Geometry: final body of the model. Coordinates: model frame, mm. Face numbers are marked on the shaded views. A direction names the side the tool comes from. Give positions to 0.01 mm unless a question says otherwise; leave off trailing zeros. Write each loop counter-clockwise with the first axis right and the second up, starting at its lowest first coordinate (ties: lowest second). Pieces come first, ordered by that corner, then holes. Notation, with made-up numbers: (-10, 83) - (4, 83) arc R14 cw to (4, 103) - close; hole circle Ø5 at (-10.5, 24). An arc over 180 degrees is marked (long way). Use CSV: the item, a comma, the result in double quotes. Start each with the question number.
(1) Section D-D on y = 220. Output: boundary loops of the cut face in (x, z), and give its area (3 significant figures).
(2) Section B-B on z = 62. Output: boundary loops of the cut face in (x, y).
(3) Line query: probe 1 along Z at (x, y) = (0, 14.75); probe 2 along Y at (x, z) = (0, -1); probe 3 along Y at (x, z) = (0, 2.75). Output: solid intervals per line, ascending. Write a range as [from, to].
(4) Section C-C on y = 15.5. Output: boundary loops of the cut face in (x, z).
(5) Reachability of the marked faces 1 and 2 from +Z, -Z, +X, -X, +Y, -Y: full face, straight path, thin tool, end or side. Return the list, or none.
(6) First-contact query: pin 1 Ø4 at (x, z) = (2.5, 38) entering from -Y; pin 2 Ø12 at (x, y) = (0, 182) entering from +Z; pin 3 Ø4 at (x, z) = (-4.5, 33) entering from -Y; pin 4 Ø10 at (y, z) = (121.5, -1) entering from -X. Flat tips, straight axial feed; report the tip coordinate or a pass-through.
(7) Section A-A on y = 100. Output: boundary loops of the cut face in (x, z).
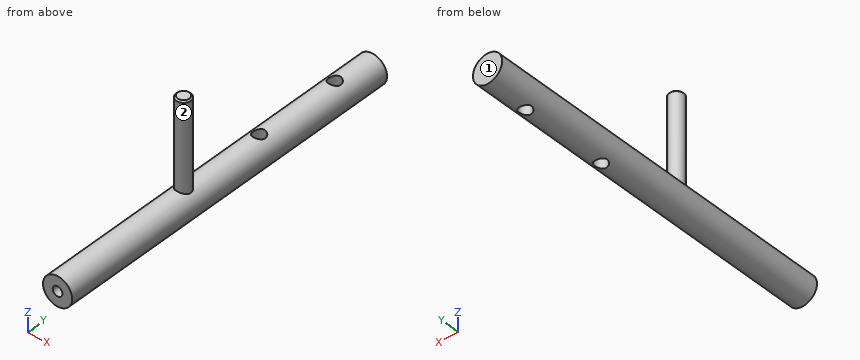
Autodesk Inventor part; units mm, degrees
ref_plane "Arbeitsebene1" through (0, 0, 3.5) normal (0, 0, 1) x (1, 0, 0)
ref_plane "YZ Plane" through (0, 0, 0) normal (1, 0, 0) x (0, 1, 0)
ref_plane "XZ Plane" through (0, 0, 0) normal (0, 1, 0) x (-1, 0, 0)
sketch "Skizze1" plane through (0, 0, 0) normal (0, 1, 0) x (-1, 0, 0)
  circle A0 centre (0, 0) radius 10
  dimension "d17" = 20
extrude "Extrusion1" add sketch "Skizze1" along normal blind 250
sketch "Skizze4" plane through (0, 0, 0) normal (0, 0, 1) x (1, 0, 0)
  line L0 (0, 0) -> (0, 100)
  circle A0 centre (0, 100) radius 5
  dimension "d10" = 100
  dimension "d11" = 10
extrude "Extrusion3" add sketch "Skizze4" along normal blind 70
ref_plane "Arbeitsebene1" through (0, 0, 3.5) normal (0, 0, 1) x (1, 0, 0)
sketch "Skizze6" plane through (0, 0, 3.5) normal (0, 0, 1) x (1, 0, 0)
  line L0 (10, 250) -> (-10, 250)
  line L1 (0, 250) -> (0, 220)
  circle A0 centre (0, 220) radius 4.25
  line L2 (0, 220) -> (0, 160)
  circle A1 centre (0, 160) radius 4.25
  point P0 (0, 0)
  dimension "d19" = 30
  dimension "d20" = 8.5
  dimension "d21" = 60
  dimension "d22" = 8.5
extrude "Extrusion5" cut sketch "Skizze6" along normal through all both and the other way through all
chamfer "Fasen1" distance 1 angle 45 1 edges at (-5, 100, 70)
thread "Gewinde2"
sketch "Skizze7" plane through (0, 0, 0) normal (0, -1, 0) x (1, 0, 0)
  point P0 (0, 0)
hole "Bohrung1" at (0, 0, 0) direction (0, 1, 0) diameter 6.647 depth 22.2 tip angle 118
properties part number "Ruderstange" material "Edelstahl"
Check values:
1,outline,"(-4.25, -9.05) - (-4.25, 9.05) arc R10 ccw to start; (4.25, -9.05) arc R10 ccw to (4.25, 9.05) - close"
1,area,"149 mm²"
2,outline,"circle Ø10 at (0, 100)"
3,probe 1,"z = [-10, -3.32], [3.32, 10]"
3,probe 2,"y = [23.6, 155.75], [164.25, 215.75], [224.25, 250]"
3,probe 3,"y = [22.54, 155.75], [164.25, 215.75], [224.25, 250]"
4,outline,"circle Ø20 at (0, 0); hole circle Ø6.65 at (0, 0)"
5,face 1,"+Z, -Z, +X, -X, +Y"
5,face 2,"+Z"
6,pin 1,"stops at y = 95.03"
6,pin 2,"stops at z = 10"
6,pin 3,"stops at y = 95.67"
6,pin 4,"stops at x = -10"
7,outline,"(-5, 8.66) arc R10 ccw (long way) to (5, 8.66) - (5, 69) - (4, 70) - (-4, 70) - (-5, 69) - close"
